Design review of the part built by this model. Coordinates are the model's own, in mm. Coordinates: 2 decimals unless noted, no trailing zeros. Loops run counter-clockwise (first coordinate to the right, second up) from the corner with the lowest first, then second, coordinate; pieces in that order, holes last. Notation, with made-up numbers: (19, -12.75) -> (54, -12.75) arc R30 ccw to (54, 26.25) -> close; hole circle Ø3 at (78, 44.5). An arc over 180 degrees is marked (long way). Use a Markdown table: item, result. Add a question column.
Q1. Take a section at C-C on x = 25. Write out the cut boundary in (y, z).
Q2. Take a section at D-D on z = -102.5. Write out the cut boundary in (x, y).
Q3. For probe 1 along X at (y, z) = (-3.5, -82.5); probe 2 along X at (y, z) = (-6.25, -102.5); probe 3 along X at (y, z) = (-8, -61.5), list the stretches that pass through material, from the lowest coordinate up.
Q4. Take a section at B-B on z = -39. Write out the cut boundary in (x, y).
Q5. Take a section at A-A on z = 63.14. Write out the cut boundary in (x, y) (3 decimals), plus the area to 3 significant figures.
Q6. Draft analysis for pull direction Z (two halves, no side actions). For faces 1 (the face through (-24.56, -4.93, 72.51)), 2 (the face through (-1, -5, 112.5)), 3 (the face through (-24.09, -5.07, -98.4)), state which applies: pulls with the +Z half, pulls with the -Z half, needs draft (parallel to the pull), parting line crosses it, or undercut.
from build123d import *

# Parameters (mm, degrees)
SKETCH1_W                      = 80
SKETCH1_H                      = 225
BOSS_EXTRUDE1_DEPTH            = 10
CUT_EXTRUDE1_REACH             = 121.818
SKETCH2_R                      = 10
M8_CLEARANCE_HOLE1_D           = 8.4
F_8_0MM_DOWEL_HOLE1_D          = 8
M6_CLEARANCE_HOLE1_D           = 6.4
M6_CLEARANCE_HOLE1_CSINK_D     = 6.45
M6_CLEARANCE_HOLE1_CSINK_ANGLE = 90


with BuildPart() as part:
    # Sketch1 → Boss-Extrude1 (new body)
    with BuildSketch(Plane(origin=(0, 0, 0), x_dir=(1, 0, 0), z_dir=(0, 1, 0))):
        Rectangle(SKETCH1_W, SKETCH1_H)
    extrude(amount=-BOSS_EXTRUDE1_DEPTH)

    # Sketch2 → Cut-Extrude1 (cut, up to next)
    with BuildSketch(Plane(origin=(0, 0, 0), x_dir=(1, 0, 0), z_dir=(0, 1, 0)), mode=Mode.PRIVATE) as cut_extrude1_sk1:
        with Locations(Location((25, -82.5, 0), (0, 0, 270))):
            Circle(SKETCH2_R)
    cut_extrude1_tool1 = extrude(cut_extrude1_sk1.sketch, amount=-CUT_EXTRUDE1_REACH, mode=Mode.PRIVATE) & part.part
    # Sketch2 → Cut-Extrude1 (cut, up to next)
    with BuildSketch(Plane(origin=(0, 0, 0), x_dir=(1, 0, 0), z_dir=(0, 1, 0)), mode=Mode.PRIVATE) as cut_extrude1_sk2:
        with Locations(Location((0, -82.5, 0), (0, 0, 270))):
            Circle(SKETCH2_R)
    cut_extrude1_tool2 = extrude(cut_extrude1_sk2.sketch, amount=-CUT_EXTRUDE1_REACH, mode=Mode.PRIVATE) & part.part
    # Sketch2 → Cut-Extrude1 (cut, up to next)
    with BuildSketch(Plane(origin=(0, 0, 0), x_dir=(1, 0, 0), z_dir=(0, 1, 0)), mode=Mode.PRIVATE) as cut_extrude1_sk3:
        with Locations(Location((-25, -82.5, 0), (0, 0, 270))):
            Circle(SKETCH2_R)
    cut_extrude1_tool3 = extrude(cut_extrude1_sk3.sketch, amount=-CUT_EXTRUDE1_REACH, mode=Mode.PRIVATE) & part.part
    # Sketch2 → Cut-Extrude1 (cut, up to next)
    with BuildSketch(Plane(origin=(0, 0, 0), x_dir=(1, 0, 0), z_dir=(0, 1, 0)), mode=Mode.PRIVATE) as cut_extrude1_sk4:
        with Locations(Location((25, -33, 0), (0, 0, 270))):
            Circle(SKETCH2_R)
    cut_extrude1_tool4 = extrude(cut_extrude1_sk4.sketch, amount=-CUT_EXTRUDE1_REACH, mode=Mode.PRIVATE) & part.part
    # Sketch2 → Cut-Extrude1 (cut, up to next)
    with BuildSketch(Plane(origin=(0, 0, 0), x_dir=(1, 0, 0), z_dir=(0, 1, 0)), mode=Mode.PRIVATE) as cut_extrude1_sk5:
        with Locations(Location((-25, -33, 0), (0, 0, 270))):
            Circle(SKETCH2_R)
    cut_extrude1_tool5 = extrude(cut_extrude1_sk5.sketch, amount=-CUT_EXTRUDE1_REACH, mode=Mode.PRIVATE) & part.part
    # Sketch2 → Cut-Extrude1 (cut, up to next)
    with BuildSketch(Plane(origin=(0, 0, 0), x_dir=(1, 0, 0), z_dir=(0, 1, 0)), mode=Mode.PRIVATE) as cut_extrude1_sk6:
        with Locations(Location((25, 39, 0), (0, 0, 270))):
            Circle(SKETCH2_R)
    cut_extrude1_tool6 = extrude(cut_extrude1_sk6.sketch, amount=-CUT_EXTRUDE1_REACH, mode=Mode.PRIVATE) & part.part
    # Sketch2 → Cut-Extrude1 (cut, up to next)
    with BuildSketch(Plane(origin=(0, 0, 0), x_dir=(1, 0, 0), z_dir=(0, 1, 0)), mode=Mode.PRIVATE) as cut_extrude1_sk7:
        with Locations(Location((-25, 47, 0), (0, 0, 270))):
            Circle(SKETCH2_R)
    cut_extrude1_tool7 = extrude(cut_extrude1_sk7.sketch, amount=-CUT_EXTRUDE1_REACH, mode=Mode.PRIVATE) & part.part
    # Sketch2 → Cut-Extrude1 (cut, up to next)
    with BuildSketch(Plane(origin=(0, 0, 0), x_dir=(1, 0, 0), z_dir=(0, 1, 0)), mode=Mode.PRIVATE) as cut_extrude1_sk8:
        with Locations(Location((-25, 82.5, 0), (0, 0, 270))):
            Circle(SKETCH2_R)
    cut_extrude1_tool8 = extrude(cut_extrude1_sk8.sketch, amount=-CUT_EXTRUDE1_REACH, mode=Mode.PRIVATE) & part.part
    # Sketch2 → Cut-Extrude1 (cut, up to next)
    with BuildSketch(Plane(origin=(0, 0, 0), x_dir=(1, 0, 0), z_dir=(0, 1, 0)), mode=Mode.PRIVATE) as cut_extrude1_sk9:
        with Locations(Location((0, 82.5, 0), (0, 0, 270))):
            Circle(SKETCH2_R)
    cut_extrude1_tool9 = extrude(cut_extrude1_sk9.sketch, amount=-CUT_EXTRUDE1_REACH, mode=Mode.PRIVATE) & part.part
    # Sketch2 → Cut-Extrude1 (cut, up to next)
    with BuildSketch(Plane(origin=(0, 0, 0), x_dir=(1, 0, 0), z_dir=(0, 1, 0)), mode=Mode.PRIVATE) as cut_extrude1_sk10:
        with Locations(Location((25, 82.5, 0), (0, 0, 270))):
            Circle(SKETCH2_R)
    cut_extrude1_tool10 = extrude(cut_extrude1_sk10.sketch, amount=-CUT_EXTRUDE1_REACH, mode=Mode.PRIVATE) & part.part
    add(cut_extrude1_tool1.solids().sort_by_distance((25, 0, 82.5))[0], mode=Mode.SUBTRACT)
    add(cut_extrude1_tool2.solids().sort_by_distance((0, 0, 82.5))[0], mode=Mode.SUBTRACT)
    add(cut_extrude1_tool3.solids().sort_by_distance((-25, 0, 82.5))[0], mode=Mode.SUBTRACT)
    add(cut_extrude1_tool4.solids().sort_by_distance((25, 0, 33))[0], mode=Mode.SUBTRACT)
    add(cut_extrude1_tool5.solids().sort_by_distance((-25, 0, 33))[0], mode=Mode.SUBTRACT)
    add(cut_extrude1_tool6.solids().sort_by_distance((25, 0, -39))[0], mode=Mode.SUBTRACT)
    add(cut_extrude1_tool7.solids().sort_by_distance((-25, 0, -47))[0], mode=Mode.SUBTRACT)
    add(cut_extrude1_tool8.solids().sort_by_distance((-25, 0, -82.5))[0], mode=Mode.SUBTRACT)
    add(cut_extrude1_tool9.solids().sort_by_distance((0, 0, -82.5))[0], mode=Mode.SUBTRACT)
    add(cut_extrude1_tool10.solids().sort_by_distance((25, 0, -82.5))[0], mode=Mode.SUBTRACT)

    # M8 Clearance Hole1 (through all)
    with Locations(Plane(origin=(0, 0, 0), x_dir=(1, 0, 0), z_dir=(0, 1, 0))):
        with Locations((25, -102.5), (-25, -102.5), (25, 102.5), (-25, 102.5)):
            Hole(M8_CLEARANCE_HOLE1_D / 2)

    # Ø8.0mm Dowel Hole1 (through all)
    with Locations(Plane(origin=(0, 0, 0), x_dir=(1, 0, 0), z_dir=(0, 1, 0))):
        with Locations((-9.5, -102.5), (9.5, 102.5)):
            Hole(F_8_0MM_DOWEL_HOLE1_D / 2)

    # M6 Clearance Hole1 (through all)
    with Locations(Plane(origin=(0, 0, 0), x_dir=(1, 0, 0), z_dir=(0, 1, 0))):
        with Locations((-24, -6.14), (-24, 25.86), (31.25, -11.64), (31.25, 16.36), (18.5, 61.5), (-6.5, 61.5), (6, -51.64), (6, -63.14)):
            CounterSinkHole(M6_CLEARANCE_HOLE1_D / 2, M6_CLEARANCE_HOLE1_CSINK_D / 2, counter_sink_angle=M6_CLEARANCE_HOLE1_CSINK_ANGLE)


solid = part.part
Answer list:
| question | item | result |
|---|---|---|
| 1 | outline | (-10, -112.5) -> (0, -112.5) -> (0, -106.7) -> (-10, -106.7) -> close; (-10, -98.3) -> (0, -98.3) -> (0, -92.5) -> (-10, -92.5) -> close; (-10, -72.5) -> (0, -72.5) -> (0, -49) -> (-10, -49) -> close; (-10, -29) -> (0, -29) -> (0, 23) -> (-10, 23) -> close; (-10, 43) -> (0, 43) -> (0, 72.5) -> (-10, 72.5) -> close; (-10, 92.5) -> (0, 92.5) -> (0, 98.3) -> (-10, 98.3) -> close; (-10, 106.7) -> (0, 106.7) -> (0, 112.5) -> (-10, 112.5) -> close |
| 2 | outline | (-40, -10) -> (-29.2, -10) -> (-29.2, 0) -> (-40, 0) -> close; (-20.8, -10) -> (5.5, -10) -> (5.5, 0) -> (-20.8, 0) -> close; (13.5, -10) -> (20.8, -10) -> (20.8, 0) -> (13.5, 0) -> close; (29.2, -10) -> (40, -10) -> (40, 0) -> (29.2, 0) -> close |
| 3 | probe 1 | -40 to -35, -15 to -10, 10 to 15, 35 to 40 |
| 3 | probe 2 | -40 to -29.2, -20.8 to 5.5, 13.5 to 20.8, 29.2 to 40 |
| 3 | probe 3 | -40 to -9.7, -3.3 to 15.3, 21.7 to 40 |
| 4 | outline | (-40, -10) -> (-31, -10) -> (-31, 0) -> (-40, 0) -> close; (-19, -10) -> (15, -10) -> (15, 0) -> (-19, 0) -> close; (35, -10) -> (40, -10) -> (40, 0) -> (35, 0) -> close |
| 5 | outline | (-40, -10) -> (2.8, -10) -> (2.8, -0.025) -> (2.775, 0) -> (-40, 0) -> close; (9.2, -10) -> (40, -10) -> (40, 0) -> (9.225, 0) -> (9.2, -0.025) -> close |
| 5 | area | 736 mm² |
| 6 | face 1 | undercut |
| 6 | face 2 | pulls with the +Z half |
| 6 | face 3 | undercut |
